Work out the finished part from the listing and answer in its coordinate system (mm). A direction names the side the tool comes from. Round coordinates to 2 decimals unless told otherwise and drop trailing zeros. Loops run counter-clockwise (first coordinate to the right, second up) from the corner with the lowest first, then second, coordinate; pieces in that order, holes last. Notation, with made-up numbers: (55, 75.5) - (73, 75.5) arc R31 ccw to (73, 101.5) - close; hole circle Ø2 at (89, 55). An arc over 180 degrees is marked (long way). Return JSON: item names as keys, results as strings.
from build123d import *

# Parameters (mm, degrees)
SKETCH1_W           = 32
SKETCH1_H           = 8
BOSS_EXTRUDE1_DEPTH = 4
SKETCH2_W           = 31.9
SKETCH2_H           = 7.9
BOSS_EXTRUDE2_DEPTH = 2
SKETCH4_W           = 29
SKETCH4_H           = 5
CUT_EXTRUDE2_DEPTH  = 3
CUT_EXTRUDE3_DEPTH  = 10


with BuildPart() as part:
    # Sketch1 → Boss-Extrude1 (new body)
    with BuildSketch(Plane(origin=(0, 0, 0), x_dir=(1, 0, 0), z_dir=(0, 1, 0))):
        with Locations((64.774193548, -9.096774194)):
            Rectangle(SKETCH1_W, SKETCH1_H)
    extrude(amount=BOSS_EXTRUDE1_DEPTH)

    # Sketch2 → Boss-Extrude2 (add)
    with BuildSketch(Plane(origin=(0, 4, 0), x_dir=(1, 0, 0), z_dir=(0, 1, 0))):
        with Locations((64.774193548, -9.096774194)):
            Rectangle(SKETCH2_W, SKETCH2_H)
    extrude(amount=BOSS_EXTRUDE2_DEPTH)

    # Sketch4 → Cut-Extrude2 (cut)
    with BuildSketch(Plane.XZ):
        with Locations((64.774193548, 9.096774194)):
            Rectangle(SKETCH4_W, SKETCH4_H)
    extrude(amount=-CUT_EXTRUDE2_DEPTH, mode=Mode.SUBTRACT)

    # Sketch3 → Cut-Extrude3 (cut)
    with BuildSketch(Plane(origin=(0, 0, 5.146774194), x_dir=(-1, 0, 0), z_dir=(0, 0, -1))):
        Polygon((-77.724193548, 4), (-77.079193548, 6), (-79.594193548, 6), (-78.949193548, 4), align=None)
        Polygon((-82.594193548, 6), (-81.949193548, 4), (-80.724193548, 4), (-80.079193548, 6), align=None)
        Polygon((-74.724193548, 4), (-74.079193548, 6), (-76.594193548, 6), (-75.949193548, 4), align=None)
        Polygon((-71.724193548, 4), (-71.079193548, 6), (-73.594193548, 6), (-72.949193548, 4), align=None)
        Polygon((-68.724193548, 4), (-68.079193548, 6), (-70.594193548, 6), (-69.949193548, 4), align=None)
        Polygon((-65.724193548, 4), (-65.079193548, 6), (-67.594193548, 6), (-66.949193548, 4), align=None)
        Polygon((-62.724193548, 4), (-62.079193548, 6), (-64.594193548, 6), (-63.949193548, 4), align=None)
        Polygon((-59.724193548, 4), (-59.079193548, 6), (-61.594193548, 6), (-60.949193548, 4), align=None)
        Polygon((-56.724193548, 4), (-56.079193548, 6), (-58.594193548, 6), (-57.949193548, 4), align=None)
        Polygon((-53.724193548, 4), (-53.079193548, 6), (-55.594193548, 6), (-54.949193548, 4), align=None)
        Polygon((-50.724193548, 4), (-50.079193548, 6), (-52.594193548, 6), (-51.949193548, 4), align=None)
        Polygon((-47.724193548, 4), (-47.079193548, 6), (-49.594193548, 6), (-48.949193548, 4), align=None)
        Polygon((-44.724193548, 4), (-44.079193548, 6), (-46.594193548, 6), (-45.949193548, 4), align=None)
    extrude(amount=-CUT_EXTRUDE3_DEPTH, mode=Mode.SUBTRACT)


solid = part.part
1) Section B-B (x = 66) is taken. Give the vertices of the cut face in (y, z).
Verdict:
{"outline": "(0, 5.1) - (4, 5.1) - (4, 13.1) - (0, 13.1) - (0, 11.6) - (3, 11.6) - (3, 6.6) - (0, 6.6) - close"}
2) Determine the mould class of faces 4 (the flat face through (65.4, 5, 9)), 5 (the flat face through (48.774, 2, 9)), 6 (the flat face through (56, 5, 5.147)) for opening direction X: pulls with the +X half, pulls with the -X half, needs draft (parallel to the pull), parting line crosses it, or undercut.
Verdict:
{"face 4": "undercut", "face 5": "pulls with the -X half", "face 6": "needs draft"}
3) Section A-A (y = 1) is taken. Give the vertices of the cut face in (x, z), and give its area (3 significant figures).
Verdict:
{"outline": "(48.77, 5.1) - (80.77, 5.1) - (80.77, 13.1) - (48.77, 13.1) - close; hole (50.27, 6.6) - (79.27, 6.6) - (79.27, 11.6) - (50.27, 11.6) - close", "area": "111 mm2"}
4) Flat-ended cylindrical pins translate along their axes: pin 1 (1.4 mm diameter, centred on x = 55.5, y = 5, fed in from -Z); pin 2 (0.5 mm diameter, centred on x = 71, y = 5, fed in from +Z); pin 3 (1.5 mm diameter, centred on x = 67.5, z = 8, fed in from -Y). Find the tip coordinate at first contact, or state that the pin passes through.
Verdict:
{"pin 1": "stops at z = 5.15", "pin 2": "stops at z = 13.05", "pin 3": "stops at y = 3"}
5) A tool of negligible diameter and unlimited length cuts with its end or side. For faces 1 (the flat face through (50, 5, 13.047)), 2 (the flat face through (68, 5, 5.147)), 3 (the flat face through (77.4, 5, 9)), from which of +Z, -Z, +X, -X, +Y, -Y can it reach the whole face along a straight path? Write none if from no direction.
Verdict:
{"face 1": "+Z, +X, -X, +Y", "face 2": "-Z, +X, -X, +Y", "face 3": "+Z, -Z, +Y"}
6) Find the intervals of material crossed by L1, parallel to X at y = 2.5, z = 9.25; L2, parallel to Z at x = 53, y = 1.25; L3, parallel to Y at x = 53, z = 9.5, in increasing order.
Verdict:
{"L1": "x = 48.77 to 50.27, 79.27 to 80.77", "L2": "z = 5.1 to 6.6, 11.6 to 13.1", "L3": "y = 3 to 6"}
